The model under review builds one solid part; all positions refer to its coordinate system, in mm. Face numbers are marked on the shaded views. A direction names the side the tool comes from. Coordinates: 2 decimals unless noted, no trailing zeros. Order: outer loops, then holes, each group sorted by start corner. A loop starts at its lowest first (then second) coordinate and runs counter-clockwise, first axis right, second up.
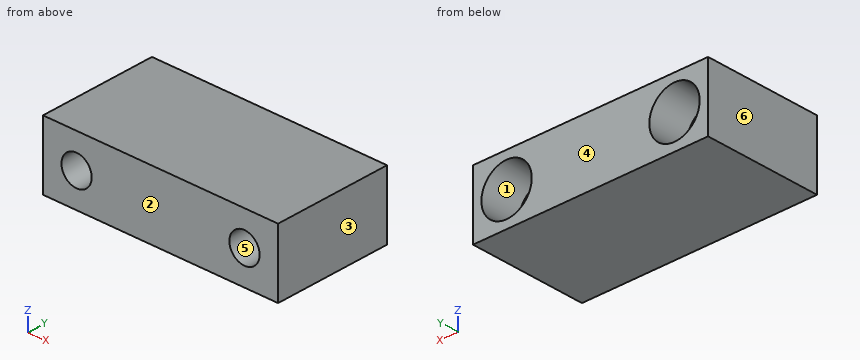
```python
from build123d import *

# Parameters (mm, degrees)
SKETCH_1_W                = 70
SKETCH_1_H                = 35
EXTRUDE_1_DEPTH           = 10
HOLE_WIZARD_1_D           = 9
HOLE_WIZARD_1_CBORE_D     = 15
HOLE_WIZARD_1_CBORE_DEPTH = 12


with BuildPart() as part:
    # 草图1 → 凸台-拉伸1 (new body, symmetric)
    with BuildSketch(Plane.XY):
        Rectangle(SKETCH_1_W, SKETCH_1_H)
    extrude(amount=EXTRUDE_1_DEPTH, both=True)

    # 打孔尺寸(%根据)内六角圆柱头螺钉的类型1 (through all)
    with Locations(Plane(origin=(-25, 17.5, 0), x_dir=(0, 0, 1), z_dir=(0, 1, 0))):
        with Locations((0, 0), (0, 50)):
            CounterBoreHole(HOLE_WIZARD_1_D / 2, HOLE_WIZARD_1_CBORE_D / 2, HOLE_WIZARD_1_CBORE_DEPTH)


solid = part.part
```
(1) We need section C-C, the plane y = 14.5. Write out the cut boundary in (x, z).
A:
outline: (-35, -10) - (35, -10) - (35, 10) - (-35, 10) - close; hole circle Ø15 at (-25, 0); hole circle Ø15 at (25, 0)
(2) We need section A-A, the plane x = -25. Write out the cut boundary in (y, z), and give its area (3 significant figures).
A:
outline: (-17.5, -10) - (17.5, -10) - (17.5, -7.5) - (5.5, -7.5) - (5.5, -4.5) - (-17.5, -4.5) - close; (-17.5, 4.5) - (5.5, 4.5) - (5.5, 7.5) - (17.5, 7.5) - (17.5, 10) - (-17.5, 10) - close
area: 313 mm2
(3) Wall thickness on probe 1 along X at (y, z) = (-4.5, 0); probe 2 along X at (y, z) = (14.25, 0); probe 3 along Z at (x, y) = (27.5, -11): over which ranges is each line inside the solid? List them lowest first.
A:
probe 1: x = -35 to -29.5, -20.5 to 20.5, 29.5 to 35
probe 2: x = -35 to -32.5, -17.5 to 17.5, 32.5 to 35
probe 3: z = -10 to -3.74, 3.74 to 10
(4) We need section D-D, the plane y = -2.5. Write out the cut boundary in (x, z), and give its area (3 significant figures).
A:
outline: (-35, -10) - (35, -10) - (35, 10) - (-35, 10) - close; hole circle Ø9 at (-25, 0); hole circle Ø9 at (25, 0)
area: 1,270 mm2
(5) For pin 1 Ø4.5 at (x, z) = (24.5, 3.5) entering from +Y, flat-tipped, find the tip position at first contact; note if it passes through.
A:
pin 1: stops at y = 5.5
(6) Draft analysis for pull direction X (two halves, no side actions). For the marked faces 3, 4, 5 and 6, state which applies: released by +X, released by -X, zero draft, split by the parting line, or undercut.
A:
face 3: released by +X
face 4: zero draft
face 5: undercut
face 6: released by -X
(7) We need section B-B, the plane z = 0. Write out the cut boundary in (x, y), and give its area (3 significant figures).
A:
outline: (-35, -17.5) - (-29.5, -17.5) - (-29.5, 5.5) - (-32.5, 5.5) - (-32.5, 17.5) - (-35, 17.5) - close; (-20.5, -17.5) - (20.5, -17.5) - (20.5, 5.5) - (17.5, 5.5) - (17.5, 17.5) - (-17.5, 17.5) - (-17.5, 5.5) - (-20.5, 5.5) - close; (29.5, -17.5) - (35, -17.5) - (35, 17.5) - (32.5, 17.5) - (32.5, 5.5) - (29.5, 5.5) - close
area: 1,680 mm2
(8) Machinability: for the marked faces 1 and 2, which of the approach directions +Z, -Z, +X, -X, +Y, -Y give a long, thin tool a straight path to every point of the face, cutting with its end or side? Answer none if there is none.
A:
face 1: +Y
face 2: +Z, -Z, +X, -X, -Y
